from build123d import *

# Parameters (mm, degrees)
REVOLVE1_ANGLE                  = 180
SKETCH3_R                       = 33.02
BOSS_EXTRUDE1_DEPTH             = 38.1
SHELL1_T                        = -4.7625
CUT_EXTRUDE1_DEPTH              = 61.26815743
CUT_EXTRUDE1_DEPTH_BACK         = 61.26815743
SKETCH4_R                       = 8.255
BOSS_EXTRUDE4_REACH             = 62.268
BOSS_EXTRUDE4_END_RADIUS        = 28.2575
SKETCH5_W                       = 46.08
SKETCH5_H                       = 30.66
SKETCH5_W_2                     = 41
SKETCH5_H_2                     = 20.5
BOSS_EXTRUDE4_DIRECTION_2_DEPTH = 19.05
BOSS_EXTRUDE6_REACH             = 77.786
SKETCH8_W                       = 33.216329336
SKETCH8_H                       = 20.5
SKETCH9_W                       = 5.08
SKETCH9_H                       = 20.5
CUT_EXTRUDE2_DEPTH              = 7.5
SKETCH15_W                      = 3.063670664
SKETCH15_H                      = 20.5
SKETCH15_W_2                    = 7.783670664
CUT_EXTRUDE5_DEPTH              = 76.786126205
SKETCH10_W                      = 10.16
SKETCH10_H                      = 3.81
CUT_EXTRUDE3_DEPTH              = 70.942302745
SKETCH11_W                      = 7.62
SKETCH11_H                      = 12.7
CUT_EXTRUDE4_DEPTH              = 36.83
SKETCH16_W                      = 5.08
SKETCH16_H                      = 5.08
CUT_EXTRUDE6_DEPTH              = 40.64
SKETCH17_W                      = 22.86
SKETCH17_H                      = 6.35
CUT_EXTRUDE7_DEPTH              = 3.81
SKETCH18_W                      = 5.08
SKETCH18_H                      = 12.155
CUT_EXTRUDE8_DEPTH              = 3.81
FILLET1_R                       = 5.08


with BuildPart() as part:
    # Sketch2 → Revolve1 (revolve)
    with BuildSketch(Plane(origin=(0, 0, 0), x_dir=(1, 0, 0), z_dir=(0, 1, 0))):
        with BuildLine():
            Line((-33.02, 0), (33.02, 0))
            ThreePointArc((33.02, 0), (0, 33.02), (-33.02, 0))
        make_face()
    revolve(axis=Axis((-33.02, 0, 0), (1, 0, 0)), revolution_arc=REVOLVE1_ANGLE)

    # Sketch3 → Boss-Extrude1 (add)
    with BuildSketch(Plane.XZ):
        with Locations(Location((0, 0, 0), (0, 0, 90))):
            Circle(SKETCH3_R)
    extrude(amount=BOSS_EXTRUDE1_DEPTH)

    # Shell1
    shell1_openings = [part.faces().sort_by_distance(p)[0] for p in [
        (0, -38.1, 0),
    ]]
    offset(amount=SHELL1_T, openings=shell1_openings, kind=Kind.INTERSECTION)

    # Sketch4 → Cut-Extrude1 (cut, two sides: drawn at the far end of the back side and taken through both)
    with BuildSketch(Plane(origin=(0, 0, 0), x_dir=(0, 0, -1), z_dir=(1, 0, 0)).offset(-CUT_EXTRUDE1_DEPTH_BACK)):
        Circle(SKETCH4_R)
    extrude(amount=CUT_EXTRUDE1_DEPTH + CUT_EXTRUDE1_DEPTH_BACK, mode=Mode.SUBTRACT)

    # Boss-Extrude4: up to this sphere (the profile starts inside it)
    boss_extrude4_end = Location((0, 0, 0)) * Sphere(BOSS_EXTRUDE4_END_RADIUS, mode=Mode.PRIVATE)
    # Sketch5 → Boss-Extrude4 (add, up to the surface)
    with BuildSketch(Plane(origin=(0, 0, 0), x_dir=(1, 0, 0), z_dir=(0, 1, 0)), mode=Mode.PRIVATE) as boss_extrude4_sk1:
        with Locations((2.36, 0)):
            Rectangle(SKETCH5_W, SKETCH5_H)
        with Locations((2.36, 0)):
            Rectangle(SKETCH5_W_2, SKETCH5_H_2, mode=Mode.SUBTRACT)
    boss_extrude4_tool1 = extrude(boss_extrude4_sk1.sketch, amount=BOSS_EXTRUDE4_REACH, mode=Mode.PRIVATE) & boss_extrude4_end
    add(boss_extrude4_tool1.solids().sort_by_distance((2.36, 0, -14.77652))[0])

    # Sketch5 → Boss-Extrude4 direction 2 (add)
    with BuildSketch(Plane(origin=(0, 0, 0), x_dir=(1, 0, 0), z_dir=(0, 1, 0))):
        with Locations((2.36, 0)):
            Rectangle(SKETCH5_W, SKETCH5_H)
        with Locations((2.36, 0)):
            Rectangle(SKETCH5_W_2, SKETCH5_H_2, mode=Mode.SUBTRACT)
    extrude(amount=-BOSS_EXTRUDE4_DIRECTION_2_DEPTH)

    # Sketch8 → Boss-Extrude6 (add, up to next)
    with BuildSketch(Plane(origin=(0, 21.59, 0), x_dir=(1, 0, 0), z_dir=(0, 1, 0)), mode=Mode.PRIVATE) as boss_extrude6_sk1:
        with Locations((-1.531835332, 0)):
            Rectangle(SKETCH8_W, SKETCH8_H)
    boss_extrude6_tool1 = extrude(boss_extrude6_sk1.sketch, amount=BOSS_EXTRUDE6_REACH, mode=Mode.PRIVATE) - part.part
    add(boss_extrude6_tool1.solids().sort_by_distance((-1.531835, 21.59, 0))[0])

    # Sketch9 → Cut-Extrude2 (cut)
    with BuildSketch(Plane.XZ.offset(-21.59)):
        with Locations((-7.345, 0)):
            Rectangle(SKETCH9_W, SKETCH9_H)
    extrude(amount=-CUT_EXTRUDE2_DEPTH, mode=Mode.SUBTRACT)

    # Sketch15 → Cut-Extrude5 (cut, through all)
    with BuildSketch(Plane.XZ.offset(-21.59)):
        with Locations((-16.608164668, 0)):
            Rectangle(SKETCH15_W, SKETCH15_H)
        with Locations((18.968164668, 0)):
            Rectangle(SKETCH15_W_2, SKETCH15_H)
    extrude(amount=CUT_EXTRUDE5_DEPTH, mode=Mode.SUBTRACT)

    # Sketch10 → Cut-Extrude3 (cut, through all)
    with BuildSketch(Plane.XZ.offset(19.05)):
        with Locations((0, -19.775)):
            Rectangle(SKETCH10_W, SKETCH10_H)
    extrude(amount=-CUT_EXTRUDE3_DEPTH, mode=Mode.SUBTRACT)

    # Sketch11 → Cut-Extrude4 (cut)
    with BuildSketch(Plane.XZ.offset(19.05)):
        with Locations((-21.95, 0)):
            Rectangle(SKETCH11_W, SKETCH11_H)
    extrude(amount=-CUT_EXTRUDE4_DEPTH, mode=Mode.SUBTRACT)

    # Sketch16 → Cut-Extrude6 (cut)
    with BuildSketch(Plane(origin=(0, -19.05, 0), x_dir=(-1, 0, 0), z_dir=(0, -1, 0))):
        with Locations((0, 12.79)):
            Rectangle(SKETCH16_W, SKETCH16_H)
    extrude(amount=-CUT_EXTRUDE6_DEPTH, mode=Mode.SUBTRACT)

    # Sketch17 → Cut-Extrude7 (cut)
    with BuildSketch(Plane.XZ.offset(-21.59)):
        with Locations((8.89, 0)):
            Rectangle(SKETCH17_W, SKETCH17_H)
    extrude(amount=-CUT_EXTRUDE7_DEPTH, mode=Mode.SUBTRACT)

    # Sketch18 → Cut-Extrude8 (cut)
    with BuildSketch(Plane.XZ.offset(-21.59)):
        with Locations((0, -9.2525)):
            Rectangle(SKETCH18_W, SKETCH18_H)
    extrude(amount=-CUT_EXTRUDE8_DEPTH, mode=Mode.SUBTRACT)

    # Fillet1
    fillet1_edges = [part.edges().sort_by_distance(p)[0] for p in [
        (-2.54, 23.495, 3.175),
        (2.54, 23.495, -3.175),
    ]]
    fillet(fillet1_edges, radius=FILLET1_R)


solid = part.part
Source: CAD feature listing. Evaluate the final solid. Frame: model axes, mm. A direction names the side the tool comes from. Coordinates: 2 decimals unless noted, no trailing zeros. Loops run counter-clockwise (first coordinate to the right, second up) from the corner with the lowest first, then second, coordinate; pieces in that order, holes last. Notation, with made-up numbers: (-39.75, -10.5) - (6.25, -10.5) arc R26 ccw to (6.25, 27.5) - close; hole circle Ø9 at (23, 2.25). An arc over 180 degrees is marked (long way). Return JSON: item names as keys, results as strings.
Q1. Section C-C, the plane z = 0. Give the number of separate pieces and of enclosed holes in the cut face, plus the area to 3 significant figures.
Results:
{"separate pieces": "3", "enclosed holes": "0", "area": "777 mm2"}
Q2. Material intervals for line 1 along X through (y, z) = (-13, 0); line 2 along X through (y, z) = (22.5, -0.5) (3 decimals); line 3 along X through (y, z) = (16, 6), sorted ascending.
Results:
{"line 1": "-33.02 to -28.26, 22.86 to 25.4, 28.26 to 33.02", "line 2": "-24.162 to -9.885, -4.805 to -2.342, 20.32 to 24.162", "line 3": "-28.25 to -25.76, 22.86 to 28.25"}
Q3. Mould query, pull axis X, two halves, no side actions, for faces 5 (the flat face through (-14.8, -38.1, 24.3)), 6 (the flat face through (-18.14, 2, 7)). Classes: released by +X, released by -X, zero draft, split by the parting line, or undercut.
Results:
{"face 5": "zero draft", "face 6": "undercut"}
Q4. Section B-B, the plane y = 2.5. Return loops of the section in (x, z), plus the area to 3 significant figures.
Results:
{"outline": "(-31.97, -7.87) arc R32.93 ccw to (31.97, -7.87) - (27.02, -7.87) arc R28.15 cw to (25.4, -12.13) - (25.4, 12.13) arc R28.15 cw to (27.02, 7.87) - (31.97, 7.87) arc R32.93 ccw to (-31.97, 7.87) - (-27.02, 7.87) arc R28.15 cw to (23.61, 15.33) - (-20.68, 15.33) - (-20.68, 6.35) - (-18.14, 6.35) - (-18.14, 10.25) - (22.86, 10.25) - (22.86, -10.25) - (2.54, -10.25) - (2.54, -15.33) - (23.61, -15.33) arc R28.15 cw to (-27.02, -7.87) - close; (-20.68, -15.33) - (-2.54, -15.33) - (-2.54, -10.25) - (-18.14, -10.25) - (-18.14, -6.35) - (-20.68, -6.35) - close", "area": "1,270 mm2"}
Q5. Access query for faces 1 (the flat face through (5.08, 22, -20)), 2 (the cylindrical face through (29.989, -3.162, -7.626)), 3 (the flat face through (13, 3, -15.33)), 4 (the cylindrical face through (-30.073, -7.324, -3.809)). Directions: +Z, -Z, +X, -X, +Y, -Y. A direction counts if a zero-diameter tool reaches every point of the face in a straight line with its end or side. Return the directions, or none.
Results:
{"face 1": "+Y, -Y", "face 2": "+X", "face 3": "-Y", "face 4": "-X"}
Q6. Section D-D, the plane y = -30. Return loops of the section in (x, z) (1 decimal), plus the area to 3 significant figures.
Results:
{"outline": "circle Ø66 at (0, 0); hole circle Ø56.5 at (0, 0)", "area": "917 mm2"}
Q7. Contact query for flat-ended pins moving along their axis: P1, Ø1.4, axis at x = -24, z = -0.5, coming from the -Y side; P2, Ø3, axis at x = -11.5, y = 10.5, coming from the -Z side; P3, Ø2.5, axis at x = -14.5, z = -2, coming from the -Y side. Output: stop coordinate, or through.
Results:
{"P1": "y = 17.78", "P2": "z = -29.87", "P3": "y = 21.59"}
